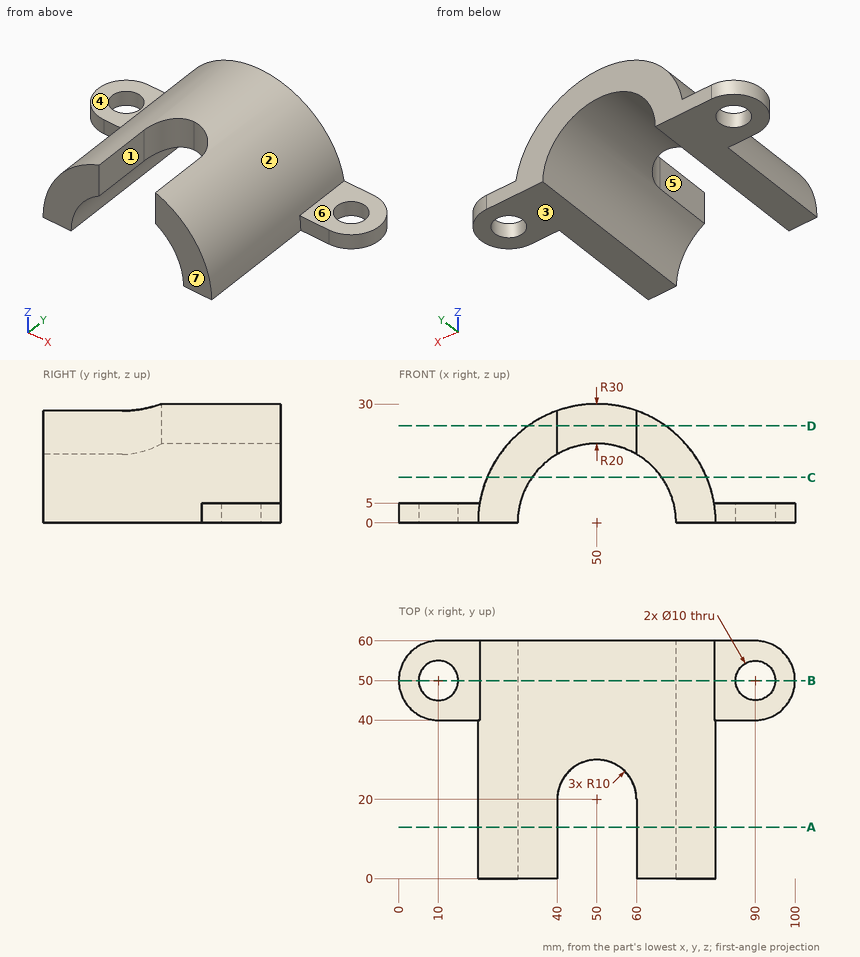
The drawing under review shows one solid part. Ordinate dimensions are in mm from its lowest x, y, z. A direction names the side the tool comes from. Give positions to 0.01 mm unless a question says otherwise; leave off trailing zeros. Loops run counter-clockwise (first coordinate to the right, second up) from the corner with the lowest first, then second, coordinate; pieces in that order, holes last. Notation, with made-up numbers: M 32,21.5 L 60,21.5 A8 cw 60,30.5 Z; hole C -38,82 d5. An arc over 180 degrees is marked long. Return JSON: item names as keys, results as strings. Group by question number.
Item 1: We need section B-B (y = 50). Give the boundary of the cut face in (x, z).
Item 2: We need section D-D (z = 24.5). Give the boundary of the cut face in (x, y), and give its area (3 significant figures).
Item 3: Mouldability with a two-part tool opening along X and no side actions: class the marked faces 1, 2 and 3 as released by +X, released by -X, zero draft, split by the parting line, or undercut.
Item 4: Insertion check: pin 1 Ø10 at (x, y) = (88, 48.5) entering from +Z; pin 2 Ø2.5 at (x, z) = (12.5, 1.5) entering from -Y; pin 3 Ø2 at (y, z) = (28.5, 25) entering from -X. Each pin has a flat end and moves straight along its axis. Give the tip position at first contact, or say it passes through.
Item 5: We need section C-C (z = 11.5). Give the boundary of the cut face in (x, y).
Item 6: For probe 1 along Y at (x, z) = (90, 3.8); probe 2 along Z at (x, y) = (82.5, 47); probe 3 along X at (y, z) = (42.5, 8), list the stretches that pass through material, from the lowest coordinate up.
Item 7: Tool access review of the marked faces 4, 5, 6 and 7: name each direction out of +Z, -Z, +X, -X, +Y, -Y from which nothing blocks a thin tool from reaching the whole face with its end or side.
Item 8: We need section A-A (y = 13). Give the boundary of the cut face in (x, z), and give its area (3 significant figures).
Output:
{
 "1": {"outline": "M 0,0 L 5,0 L 5,5 L 0,5 Z; M 15,0 L 30,0 A20 cw 70,0 L 85,0 L 85,5 L 79.58,5 A30 ccw 20.42,5 L 15,5 Z; M 95,0 L 100,0 L 100,5 L 95,5 Z"},
 "2": {"outline": "M 32.69,0 L 40,0 L 40,20 A10 cw 60,20 L 60,0 L 67.31,0 L 67.31,60 L 32.69,60 Z", "area": "1,520 mm^2"},
 "3": {"face 1": "undercut", "face 2": "split by the parting line", "face 3": "zero draft"},
 "4": {"pin 1": "stops at z = 5", "pin 2": "stops at y = 40", "pin 3": "stops at x = 32"},
 "5": {"outline": "M 22.29,0 L 33.64,0 L 33.64,60 L 22.29,60 Z; M 66.36,0 L 77.71,0 L 77.71,60 L 66.36,60 Z"},
 "6": {"probe 1": "y = 40 to 45, 55 to 60", "probe 2": "z = 0 to 5", "probe 3": "x = 21.09 to 31.67, 68.33 to 78.91"},
 "7": {"face 4": "+Z, -X, +Y, -Y", "face 5": "+Z, -Z, -Y", "face 6": "+Z, +X, +Y, -Y", "face 7": "+Z, -Z, +X, -X, -Y"},
 "8": {"outline": "M 20,0 L 30,0 A20 cw 40,17.32 L 40,28.28 A30 ccw Z; M 60,17.32 A20 cw 70,0 L 80,0 A30 ccw 60,28.28 Z", "area": "579 mm^2"}
}
